Check sheet for the modelled part. Datum: model origin and axes. Units: mm. Face numbers are marked on the shaded views. Round coordinates to 2 decimals unless told otherwise and drop trailing zeros. Loops run counter-clockwise (first coordinate to the right, second up) from the corner with the lowest first, then second, coordinate; pieces in that order, holes last. Notation, with made-up numbers: M 63.5,74.25 L 67.5,74.25 A20 cw 67.5,97.25 Z; hole C -39,63 d7. An arc over 180 degrees is marked long. Write item = value, one per line. Start each with the question number.
(1) Cross-section at B-B on x = 51. Record the boundary of the cut face in (y, z).
(2) Cross-section at C-C on y = 9. Record the boundary of the cut face in (x, z).
(3) Cross-section at D-D on x = 78.5. Record the boundary of the cut face in (y, z), plus the area to 3 significant figures.
(4) Cross-section at A-A on y = 19.5. Record the boundary of the cut face in (x, z).
(5) Scan lines: L1, parallel to Y at x = 36, z = 4.8; L2, parallel to Y at x = 94.7, z = 2.5; L3, parallel to X at y = 86, z = 3.85. Record each from-to range of solid material in increasing order. Write a range as from..to.
(6) Mould release check, pull along X, two halves, no side actions. Record for the marked faces 1 and 2: pulls with the +X half, pulls with the -X half, needs draft (parallel to the pull), parting line crosses it, or undercut.
(7) Go/stop test with flat-tipped pins: P1, Ø1.5, axis at x = 26.5, y = 42, coming from the +Z side; P2, Ø2, axis at x = 29.5, z = 4.5, coming from the -Y side; P3, Ø0.7, axis at x = 43.5, z = 4.5, coming from the +Y side. Record where each tip stops, or that it passes through.
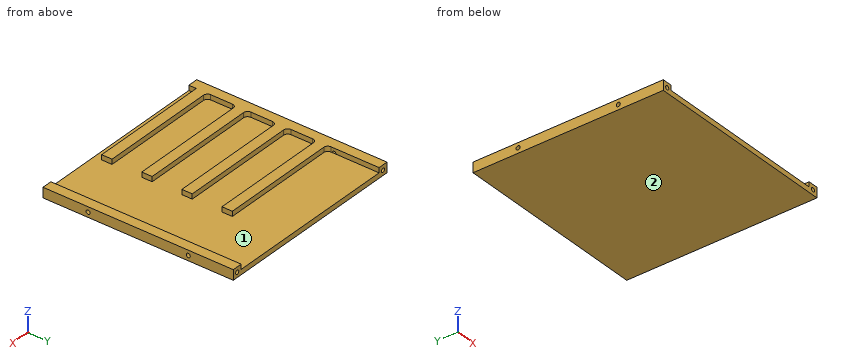
from build123d import *

# Parameters (mm, degrees)
SKETCH1_W           = 97.46
SKETCH1_H           = 97.46
BOSS_EXTRUDE1_DEPTH = 1.27
SKETCH3_W           = 5
SKETCH3_H           = 97.46
BOSS_EXTRUDE2_DEPTH = 3.73
SKETCH7_R           = 1
CUT_EXTRUDE2_DEPTH  = 5
SKETCH6_R           = 1
CUT_EXTRUDE3_DEPTH  = 5
SKETCH4_R           = 1
CUT_EXTRUDE4_DEPTH  = 5
SKETCH5_R           = 1
CUT_EXTRUDE5_DEPTH  = 5
FILLET1_R           = 2
SKETCH8_R           = 1
CUT_EXTRUDE6_DEPTH  = 10
SKETCH9_R           = 1
CUT_EXTRUDE7_DEPTH  = 10
BOSS_EXTRUDE3_DEPTH = 1.27
CUT_EXTRUDE8_DEPTH  = 1.27
CUT_EXTRUDE9_DEPTH  = 1.27


with BuildPart() as part:
    # Sketch1 → Boss-Extrude1 (new body)
    with BuildSketch(Plane.XY):
        with Locations((48.73, 48.73)):
            Rectangle(SKETCH1_W, SKETCH1_H)
    extrude(amount=BOSS_EXTRUDE1_DEPTH)

    # Sketch3 → Boss-Extrude2 (add)
    with BuildSketch(Plane.XY.offset(1.27)):
        Polygon((0, 0), (5, 0), (5, 5), (65, 5), (65, 10.172513956), (5, 10.172513956), (5, 25), (65, 25), (65, 30.172513956), (5, 30.172513956), (5, 45), (65, 45), (65, 50.172513956), (5, 50.172513956), (5, 65), (65, 65), (65, 70.172513956), (5, 70.172513956), (5, 97.46), (0, 97.46), align=None)
        with Locations((94.96, 48.73)):
            Rectangle(SKETCH3_W, SKETCH3_H)
    extrude(amount=BOSS_EXTRUDE2_DEPTH)

    # Sketch7 → Cut-Extrude2 (cut)
    with BuildSketch(Plane(origin=(0, 97.46, 0), x_dir=(-1, 0, 0), z_dir=(0, 1, 0))):
        with Locations((-2.5, 2.5)):
            Circle(SKETCH7_R)
    extrude(amount=-CUT_EXTRUDE2_DEPTH, mode=Mode.SUBTRACT)

    # Sketch6 → Cut-Extrude3 (cut)
    with BuildSketch(Plane(origin=(0, 97.46, 0), x_dir=(-1, 0, 0), z_dir=(0, 1, 0))):
        with Locations((-94.96, 2.5)):
            Circle(SKETCH6_R)
    extrude(amount=-CUT_EXTRUDE3_DEPTH, mode=Mode.SUBTRACT)

    # Sketch4 → Cut-Extrude4 (cut)
    with BuildSketch(Plane.XZ):
        with Locations((94.96, 2.5)):
            Circle(SKETCH4_R)
    extrude(amount=-CUT_EXTRUDE4_DEPTH, mode=Mode.SUBTRACT)

    # Sketch5 → Cut-Extrude5 (cut)
    with BuildSketch(Plane.XZ):
        with Locations((2.5, 2.5)):
            Circle(SKETCH5_R)
    extrude(amount=-CUT_EXTRUDE5_DEPTH, mode=Mode.SUBTRACT)

    # Fillet1
    fillet1_edges = [part.edges().sort_by_distance(p)[0] for p in [
        (5, 70.172513956, 3.135),
        (5, 50.172513956, 3.135),
        (5, 30.172513956, 3.135),
        (5, 10.172513956, 3.135),
        (5, 65, 3.135),
        (5, 45, 3.135),
        (5, 25, 3.135),
    ]]
    fillet(fillet1_edges, radius=FILLET1_R)

    # Sketch8 → Cut-Extrude6 (cut)
    with BuildSketch(Plane.ZY):
        with Locations((2.5, 23.73)):
            Circle(SKETCH8_R)
        with Locations((2.5, 73.73)):
            Circle(SKETCH8_R)
    extrude(amount=-CUT_EXTRUDE6_DEPTH, mode=Mode.SUBTRACT)

    # Sketch9 → Cut-Extrude7 (cut)
    with BuildSketch(Plane(origin=(97.46, 0, 0), x_dir=(0, 0, -1), z_dir=(1, 0, 0))):
        with Locations((-2.5, 73.73)):
            Circle(SKETCH9_R)
        with Locations((-2.5, 23.73)):
            Circle(SKETCH9_R)
    extrude(amount=-CUT_EXTRUDE7_DEPTH, mode=Mode.SUBTRACT)

    # Sketch3<5> → Boss-Extrude3 (add)
    with BuildSketch(Plane.XY.offset(1.27)):
        Polygon((65, 5), (5, 5), (5, 0), (92.46, 0), (92.46, 5), (92.46, 92.46), (92.46, 97.46), (5, 97.46), (5, 92.46), (5, 70.172513956), (65, 70.172513956), (65, 65), (5, 65), (5, 50.172513956), (65, 50.172513956), (65, 45), (5, 45), (5, 30.172513956), (65, 30.172513956), (65, 25), (5, 25), (5, 10.172513956), (65, 10.172513956), align=None)
    extrude(amount=BOSS_EXTRUDE3_DEPTH)

    # Sketch10 → Cut-Extrude8 (cut)
    with BuildSketch(Plane.XZ):
        Polygon((5, 5), (0, 5), (0, 0), (97.46, 0), (97.46, 5), (92.46, 5), (92.46, 2.54), (5, 2.54), align=None)
    extrude(amount=-CUT_EXTRUDE8_DEPTH, mode=Mode.SUBTRACT)

    # Sketch11 → Cut-Extrude9 (cut)
    with BuildSketch(Plane(origin=(0, 97.46, 0), x_dir=(1, 0, 0), z_dir=(0, 1, 0))):
        Polygon((92.46, -2.54), (92.46, -5), (97.46, -5), (97.46, 0), (0, 0), (0, -5), (5, -5), (5, -2.54), align=None)
    extrude(amount=-CUT_EXTRUDE9_DEPTH, mode=Mode.SUBTRACT)


solid = part.part
Result:
q1.outline = M 1.27,0 L 96.19,0 L 96.19,2.54 L 70.17,2.54 L 70.17,5 L 65,5 L 65,2.54 L 50.17,2.54 L 50.17,5 L 45,5 L 45,2.54 L 30.17,2.54 L 30.17,5 L 25,5 L 25,2.54 L 10.17,2.54 L 10.17,5 L 5,5 L 5,2.54 L 1.27,2.54 Z
q2.outline = M 0,0 L 97.46,0 L 97.46,5 L 92.46,5 L 92.46,2.54 L 65,2.54 L 65,5 L 0,5 Z
q3.outline = M 1.27,0 L 96.19,0 L 96.19,2.54 L 1.27,2.54 Z
q3.area = 241 mm^2
q4.outline = M 0,0 L 97.46,0 L 97.46,5 L 92.46,5 L 92.46,2.54 L 5,2.54 L 5,5 L 0,5 Z
q5.L1 = 5..10.17, 25..30.17, 45..50.17, 65..70.17
q5.L2 = 5..22.73, 24.73..72.73, 74.73..92.46
q5.L3 = 0..5, 92.46..97.46
q6.face_1 = undercut
q6.face_2 = needs draft
q7.P1 = 2.54
q7.P2 = 5
q7.P3 = 70.17
